```python
from build123d import *

# Parameters (mm, degrees)
SKETCH2_W           = 11.049
SKETCH2_H           = 1.651
SKETCH2_W_2         = 1.651
SKETCH2_H_2         = 36.449
BOSS_EXTRUDE1_DEPTH = 100


with BuildPart() as part:
    # Sketch2 → Boss-Extrude1 (new body)
    with BuildSketch(Plane.XY):
        Polygon((-12.7, 0), (-11.049, 0), (-11.049, 36.449), (-11.049, 38.1), (-12.7, 38.1), align=None)
        with Locations((-5.5245, 37.2745)):
            Rectangle(SKETCH2_W, SKETCH2_H)
        Polygon((0, 38.1), (0, 36.449), (11.049, 36.449), (11.049, 0), (12.7, 0), (12.7, 38.1), align=None)
        with Locations((11.8745, -18.2245)):
            Rectangle(SKETCH2_W_2, SKETCH2_H_2)
        Polygon((-11.049, -36.449), (-11.049, 0), (-12.7, 0), (-12.7, -38.1), (0, -38.1), (0, -36.449), align=None)
        Polygon((11.049, -36.449), (0, -36.449), (0, -38.1), (12.7, -38.1), (12.7, -36.449), align=None)
    extrude(amount=BOSS_EXTRUDE1_DEPTH)


solid = part.part
```
Build history of the part. All positions in model axes, mm. A direction names the side the tool comes from. Give positions to 0.01 mm unless a question says otherwise; leave off trailing zeros. Loops run counter-clockwise (first coordinate to the right, second up) from the corner with the lowest first, then second, coordinate; pieces in that order, holes last. Notation, with made-up numbers: (9, -32) -> (27, -32) arc R20 ccw to (27, -17) -> close; hole circle Ø10 at (75.5, 88). An arc over 180 degrees is marked (long way). One line per question, with ' | ' between items.
Q1. Tool access for faces 1 (the flat face through (-12.7, 1, 49)), 2 (the flat face through (0, 36.449, 49)): list every direction of +Z, -Z, +X, -X, +Y, -Y with a clear straight run to the whole face (end or side of a thin tool).
Filled sheet:
face 1: +Z, -Z, -X, +Y, -Y | face 2: +Z, -Z
Q2. Pull direction Y, two halves, no side cores. Call faces 3 (the flat face through (0, -38.1, 49)), 4 (the flat face through (12.7, -1, 49)), 5 (the flat face through (0, -36.449, 49)): pulls with the +Y half, pulls with the -Y half, needs draft (parallel to the pull), parting line crosses it, or undercut.
Filled sheet:
face 3: pulls with the -Y half | face 4: needs draft | face 5: undercut
Q3. Drop a flat-ended pin along its axis: pin 1 (3 mm diameter, centred on x = -8.5, y = 21, fed in from -Z). Give the stop position or say it passes through.
Filled sheet:
pin 1: passes through
Q4. Cut at A-A, the plane y = 24.5. Write the cut outline in (x, z).
Filled sheet:
outline: (-12.7, 0) -> (-11.05, 0) -> (-11.05, 100) -> (-12.7, 100) -> close; (11.05, 0) -> (12.7, 0) -> (12.7, 100) -> (11.05, 100) -> close
Q5. Cut at C-C, the plane z = 53.5. Write the cut outline in (x, y).
Filled sheet:
outline: (-12.7, -38.1) -> (12.7, -38.1) -> (12.7, 38.1) -> (-12.7, 38.1) -> close; hole (-11.05, -36.45) -> (11.05, -36.45) -> (11.05, 36.45) -> (-11.05, 36.45) -> close
Q6. Drill centre lines: line 1 along Y through (x, z) = (5.75, 80); line 2 along X through (y, z) = (-14, 25.5). Where is each one in solid material? Low to high. Write a range as [from, to].
Filled sheet:
line 1: y = [-38.1, -36.45], [36.45, 38.1] | line 2: x = [-12.7, -11.05], [11.05, 12.7]
Q7. Cut at B-B, the plane x = 3.5. Write the cut outline in (y, z).
Filled sheet:
outline: (-38.1, 0) -> (-36.45, 0) -> (-36.45, 100) -> (-38.1, 100) -> close; (36.45, 0) -> (38.1, 0) -> (38.1, 100) -> (36.45, 100) -> close
